For this review, take the finished solid that the model builds, in its own axes (mm). Coordinates: 2 decimals unless noted, no trailing zeros. Order: outer loops, then holes, each group sorted by start corner. A loop starts at its lowest first (then second) coordinate and runs counter-clockwise, first axis right, second up.
from build123d import *

# Parameters (mm, degrees)
BOSS_EXTRUDE1_DEPTH      = 214
SKETCH2_R                = 5
CUT_EXTRUDE1_DEPTH       = 222.801713249
SKETCH4_R                = 1.500000001
CUT_EXTRUDE3_DEPTH       = 222.801713249
F_3_0_3_DIAMETER_HOLE1_D = 3
F_3_0_3_DIAMETER_HOLE2_D = 3


with BuildPart() as part:
    # Sketch1 → Boss-Extrude1 (new body)
    with BuildSketch(Plane.XY):
        Polygon((0, 0), (0, 30), (2, 30), (2, 2), (50, 2), (50, 0), align=None)
    extrude(amount=BOSS_EXTRUDE1_DEPTH)

    # Sketch2 → Cut-Extrude1 (cut, through all)
    with BuildSketch(Plane.XZ):
        with Locations((14, 105)):
            Circle(SKETCH2_R)
    extrude(amount=-CUT_EXTRUDE1_DEPTH, mode=Mode.SUBTRACT)

    # Sketch4 → Cut-Extrude3 (cut, through all)
    with BuildSketch(Plane(origin=(0, 0, 0), x_dir=(-1, 0, 0), z_dir=(0, -1, 0))):
        with Locations(Location((-14.000000126, -112.999999976, 0), (0, 0, 180))):
            Circle(SKETCH4_R)
        with Locations(Location((-14.000000126, -96.999999976, 0), (0, 0, 180))):
            Circle(SKETCH4_R)
    extrude(amount=-CUT_EXTRUDE3_DEPTH, mode=Mode.SUBTRACT)

    # Ø3.0 (3) Diameter Hole1 (through all)
    with Locations(Plane(origin=(2, 0, 0), x_dir=(0, 0, -1), z_dir=(1, 0, 0))):
        with Locations((-199.5, 9.45), (-199.5, 19.45), (-184.5, 19.450012476), (-184.5, 9.45), (-29.5, 19.45), (-29.5, 9.45), (-14.5, 9.45), (-14.5, 19.45)):
            Hole(F_3_0_3_DIAMETER_HOLE1_D / 2)

    # Ø3.0 (3) Diameter Hole2 (through all)
    with Locations(Plane(origin=(-23.407632793, 2, 151.138003919), x_dir=(0, 0, 1), z_dir=(0, 1, 0))):
        with Locations((58.861996081, 61.407632793), (58.861996081, 37.407632793)):
            Hole(F_3_0_3_DIAMETER_HOLE2_D / 2)


solid = part.part
1. Take a section at B-B, the plane y = 14.5. Give the boundary of the cut face in (x, z).
Answer below:
outline: (0, 0) - (2, 0) - (2, 214) - (0, 214) - close
2. The part is to be moulded in two halves that separate along X. For faces 1 (the face through (18.77, 0.99, 106.5)), 2 (the face through (2, 16, 106)), 3 (the face through (26, 2, 106)), 4 (the face through (0, 15, 106)), say which applies: +X half, -X half, draft (parallel to the pull), parting line (faces both ways), or undercut.
Answer below:
face 1: undercut
face 2: +X half
face 3: draft
face 4: -X half
3. Take a section at A-A, the plane z = 61. Give the boundary of the cut face in (x, y).
Answer below:
outline: (0, 0) - (50, 0) - (50, 2) - (2, 2) - (2, 30) - (0, 30) - close
4. To check wall thickness, follow L1, parallel to Y at x = 0.8, z = 14.5; L2, parallel to X at y = 0.7, z = 210; L3, parallel to X at y = 1.1, z = 97. State the ranges of each line that lie inside material, in increasing order.
Answer below:
L1: y = 0 to 7.95, 10.95 to 17.95, 20.95 to 30
L2: x = 0 to 12.5, 15.5 to 36.5, 39.5 to 50
L3: x = 0 to 12.5, 15.5 to 50
5. Clearance check with flat-ended pins moving along their axes: pin 1 Ø14 at (y, z) = (22, 152.5) entering from +X; pin 2 Ø4 at (x, z) = (14, 210) entering from -Y; pin 3 Ø11.5 at (x, z) = (14, 105) entering from +Y. State where each tip first meets the part, or that it passes through.
Answer below:
pin 1: stops at x = 2
pin 2: stops at y = 0
pin 3: stops at y = 2
